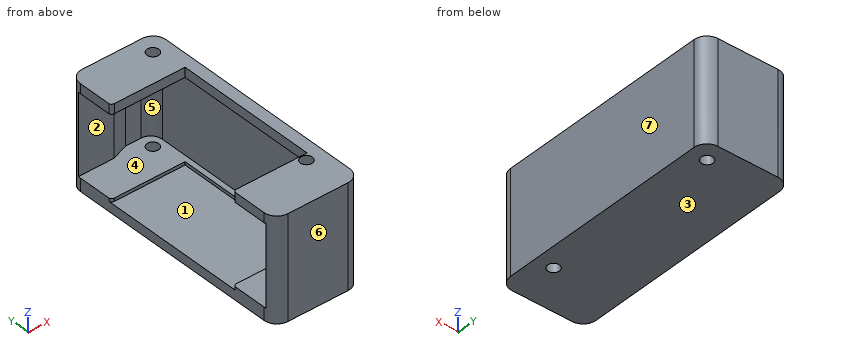
from build123d import *

# Parameters (mm, degrees)
SKETCH815_R             = 1.85
PAD351_DEPTH            = 32
POCKET_DEPTH            = 62
POCKET223_DEPTH         = 25
BODY022_PLACEMENT_ANGLE = 180


with BuildPart() as part:
    # Sketch815 → Pad351 (new body)
    with BuildSketch(Plane.XY):
        with BuildLine():
            Line((-1.610327, 37.5), (17.110638, 37.5))
            ThreePointArc((21.110638, 33.5), (19.939065, 36.328427), (17.110638, 37.5))
            Line((21.110638, 33.5), (21.110638, -33.5))
            ThreePointArc((17.110638, -37.5), (19.939065, -36.328427), (21.110638, -33.5))
            Line((17.110638, -37.5), (-1.610327, -37.5))
            ThreePointArc((-5.610327, -33.5), (-4.438754, -36.328427), (-1.610327, -37.5))
            Line((-5.610327, -33.5), (-5.610327, 33.5))
            ThreePointArc((-1.610327, 37.5), (-4.438754, 36.328427), (-5.610327, 33.5))
        make_face()
        with Locations((0, 24.3)):
            Circle(SKETCH815_R, mode=Mode.SUBTRACT)
        with Locations((0, -31.7)):
            Circle(SKETCH815_R, mode=Mode.SUBTRACT)
    extrude(amount=PAD351_DEPTH)

    # Sketch816 → Pocket (cut)
    with BuildSketch(Plane.XY.offset(65)):
        with BuildLine():
            Line((-1.941559, 22.241577), (20.093479, 22.241577))
            ThreePointArc((20.093479, 22.241577), (20.864733, 22.561041), (21.184197, 23.332295))
            Line((21.184197, 23.332295), (21.184197, 25.813278))
            Line((21.184197, 25.813278), (30.338089, 25.813278))
            Line((30.338089, 25.813278), (30.338089, 22.183402))
            Line((30.338089, 22.183402), (30.338089, -22.183402))
            Line((30.338089, -26.656548), (30.338089, -22.183402))
            Line((21.144989, -26.656548), (30.338089, -26.656548))
            Line((21.144989, -23.239975), (21.144989, -26.656548))
            ThreePointArc((21.144989, -23.239975), (20.852565, -22.534001), (20.146591, -22.241577))
            Line((20.146591, -22.241577), (-1.941559, -22.241577))
            Line((-1.941559, -22.241577), (-1.941559, 22.241577))
        make_face()
    extrude(amount=-POCKET_DEPTH, mode=Mode.SUBTRACT)

    # Sketch817 → Pocket223 (cut)
    with BuildSketch(Plane.XY.offset(4)):
        with BuildLine():
            Line((0, 36.1), (4.759236, 36.1))
            Line((4.759236, 36.1), (10.017961, 34.208318))
            Line((10.017961, 34.208318), (31.19193, 34.208318))
            Line((31.19193, 34.208318), (31.19193, -34.208318))
            Line((10.017961, -34.208318), (31.19193, -34.208318))
            Line((4.759236, -36.1), (10.017961, -34.208318))
            Line((4.759236, -36.1), (0, -36.1))
            ThreePointArc((-3.6, -32.5), (-2.545584, -35.045584), (0, -36.1))
            Line((-3.6, -32.5), (-3.6, 32.5))
            ThreePointArc((0, 36.1), (-2.545584, 35.045584), (-3.6, 32.5))
        make_face()
    extrude(amount=POCKET223_DEPTH, mode=Mode.SUBTRACT)


with BuildPart() as part_1:
    # Body022 placement: moved
    add(part.part.moved(Location((218, -96, -111))).rotate(Axis((218, -96, -111), (0, 0, 1)), BODY022_PLACEMENT_ANGLE))


solid = part_1.part
Read the model definition and answer for the solid it produces. Units are mm, in the model's axes. Face numbers are marked on the shaded views. A direction names the side the tool comes from. Round coordinates to 2 decimals unless told otherwise and drop trailing zeros. Order: outer loops, then holes, each group sorted by start corner. A loop starts at its lowest first (then second) coordinate and runs counter-clockwise, first axis right, second up.
1) For the marked faces 1, 2 and 3, determine the directions among +Z, -Z, +X, -X, +Y, -Y from which every point of the face is accessible in a straight line to the end or side of a thin tool.
2) The part is cut by section C-C on x = 206.25. Write down the section's boundary in (y, z), plus the area to 3 significant figures.
3) The part is cut by section B-B on z = -88. Write down the section's boundary in (x, y).
4) Flat-ended cylindrical pins translate along their axes: pin 1 (5 mm diameter, centred on x = 203.5, y = -106, fed in from +Z); pin 2 (12.5 mm diameter, centred on y = -92, z = -95.5, fed in from -X); pin 3 (2.5 mm diameter, centred on y = -96.5, z = -80, fed in from -X). Find the tip coordinate at first contact, or state that the pin passes through.
5) The part is cut by section A-A on y = -120.3. Write down the section's boundary in (x, z).
6) The mould has two halves that part along Y. Classify the marked faces 4, 5, 6 and 7: released by +Y, released by -Y, zero draft, split by the parting line, or undercut.
7) Straight lines are drawn through the part: L1, parallel to Y at x = 218, z = -108.25; L2, parallel to Y at x = 218, z = -107.95; L3, parallel to X at y = -120.3, z = -80.2. For each, find the intervals that lie inside material, in ascending order.
Resolved:
1. face 1: +Z, -X
1. face 2: -X
1. face 3: -Z, +X, -X, +Y, -Y
2. outline: (-133.5, -111) - (-58.5, -111) - (-58.5, -79) - (-73.76, -79) - (-73.76, -82) - (-61.79, -82) - (-61.79, -107) - (-73.76, -107) - (-73.76, -108) - (-118.24, -108) - (-118.24, -107) - (-130.21, -107) - (-130.21, -82) - (-118.24, -82) - (-118.24, -79) - (-133.5, -79) - close
2. area: 512 mm2
3. outline: (196.95, -130.21) arc R4 ccw to (200.89, -133.5) - (219.61, -133.5) arc R4 ccw to (223.61, -129.5) - (223.61, -62.5) arc R4 ccw to (219.61, -58.5) - (200.89, -58.5) arc R4 ccw to (196.95, -61.79) - (207.98, -61.79) - (213.24, -59.9) - (218, -59.9) arc R3.6 cw to (221.6, -63.5) - (221.6, -128.5) arc R3.6 cw to (218, -132.1) - (213.24, -132.1) - (207.98, -130.21) - close
4. pin 1: stops at z = -108
4. pin 2: stops at x = 221.6
4. pin 3: stops at x = 219.94
5. outline: (196.89, -111) - (216.15, -111) - (216.15, -107) - (196.89, -107) - close; (196.89, -82) - (216.15, -82) - (216.15, -79) - (196.89, -79) - close; (219.85, -111) - (223.61, -111) - (223.61, -79) - (219.85, -79) - (219.85, -82) - (221.6, -82) - (221.6, -107) - (219.85, -107) - close
6. face 4: undercut
6. face 5: undercut
6. face 6: released by -Y
6. face 7: zero draft
7. L1: y = -133.5 to -122.15, -118.45 to -66.15, -62.45 to -58.5
7. L2: y = -133.5 to -122.15, -118.45 to -118.24, -73.76 to -66.15, -62.45 to -58.5
7. L3: x = 196.89 to 216.15, 219.85 to 223.61
